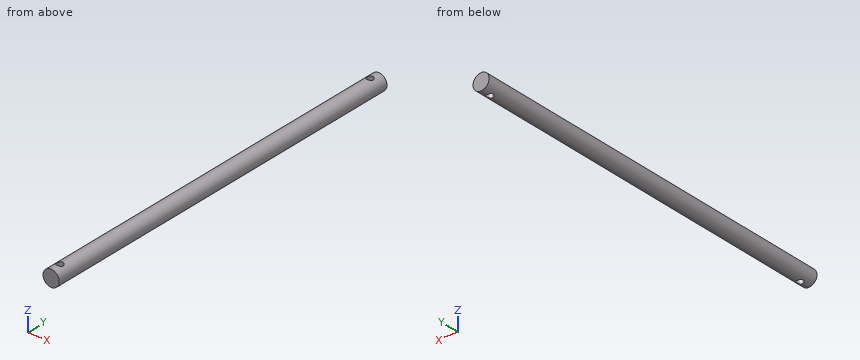
from build123d import *

# Parameters (mm, degrees)
CROQUIS1_R                 = 5
SALIENTE_EXTRUIR1_DEPTH    = 339
CROQUIS2_R                 = 6.894742802
CORTAR_EXTRUIR1_DEPTH      = 99.5
CORTAR_EXTRUIR2_DEPTH      = 10
CORTAR_EXTRUIR2_DEPTH_BACK = 10
CROQUIS3_R                 = 2
CORTAR_EXTRUIR3_DEPTH      = 10
CORTAR_EXTRUIR3_DEPTH_BACK = 10
CROQUIS4_R                 = 2


with BuildPart() as part:
    # Croquis1 → Saliente-Extruir1 (new body)
    with BuildSketch(Plane(origin=(0, 0, 0), x_dir=(1, 0, 0), z_dir=(0, 1, 0))):
        with Locations(Location((0, 0, 0), (0, 0, 270))):
            Circle(CROQUIS1_R)
    extrude(amount=SALIENTE_EXTRUIR1_DEPTH)

    # Croquis2 → Cortar-Extruir1 (cut)
    with BuildSketch(Plane(origin=(0, 339, 0), x_dir=(1, 0, 0), z_dir=(0, 1, 0))):
        Circle(CROQUIS2_R)
    extrude(amount=-CORTAR_EXTRUIR1_DEPTH, mode=Mode.SUBTRACT)

    # Croquis3 → Cortar-Extruir2 (cut, two sides: drawn at the far end of the back side and taken through both)
    with BuildSketch(Plane.XY.offset(-CORTAR_EXTRUIR2_DEPTH_BACK)):
        with Locations(Location((0, 6.5, 0), (0, 0, 90.000000001))):
            Circle(CROQUIS3_R)
    extrude(amount=CORTAR_EXTRUIR2_DEPTH + CORTAR_EXTRUIR2_DEPTH_BACK, mode=Mode.SUBTRACT)

    # Croquis4 → Cortar-Extruir3 (cut, two sides: drawn at the far end of the back side and taken through both)
    with BuildSketch(Plane.XY.offset(-CORTAR_EXTRUIR3_DEPTH_BACK)):
        with Locations(Location((0, 233, 0), (0, 0, 90.000000001))):
            Circle(CROQUIS4_R)
    extrude(amount=CORTAR_EXTRUIR3_DEPTH + CORTAR_EXTRUIR3_DEPTH_BACK, mode=Mode.SUBTRACT)


solid = part.part
Input: part model. Units: mm. Frame: model coordinates. Coordinates: 2 decimals unless noted, no trailing zeros. Write each loop counter-clockwise with the first axis right and the second up, starting at its lowest first coordinate (ties: lowest second). Pieces come first, ordered by that corner, then holes. Notation, with made-up numbers: M -3,-32.75 L 8,-32.75 A16 cw 8,-2.75 Z; hole C 44.5,-1.75 d4. An arc over 180 degrees is marked long. Answer as a JSON object with one key per item and string values. Group by question number.
(1) Section B-B on z = 2. Output: boundary loops of the cut face in (x, y), plus the area to 3 significant figures.
(2) Contact query for flat-ended pins moving along their axis: P1, Ø2, axis at x = 4, y = 76, coming from the +Z side; P2, Ø3.5, axis at x = 0, y = 233, coming from the -Z side; P3, Ø1, axis at x = 1.5, y = 197, coming from the +Z side. Output: stop coordinate, or through.
(3) Ray query, line 1 along Y through (x, z) = (0, 1.5); line 2 along Y through (x, z) = (0.5, -3); line 3 along Z through (x, y) = (0.5, 126). Return the intervals inside material, ascending. Write a range as [from, to].
(4) Section A-A on x = 0. Output: boundary loops of the cut face in (y, z), plus the area to 4 significant figures.
(5) Section C-C on y = 116. Output: boundary loops of the cut face in (x, z).
(6) Section D-D on y = 233. Output: boundary loops of the cut face in (x, z).
Result set:
{
 "1": {"outline": "M -4.58,0 L 4.58,0 L 4.58,239.5 L -4.58,239.5 Z; hole C 0,6.5 d4; hole C 0,233 d4", "area": "2,170 mm2"},
 "2": {"P1": "stops at z = 4", "P2": "passes through", "P3": "stops at z = 4.9"},
 "3": {"line 1": "y = [0, 4.5], [8.5, 231], [235, 239.5]", "line 2": "y = [0, 4.56], [8.44, 231.06], [234.94, 239.5]", "line 3": "z = [-4.97, 4.97]"},
 "4": {"outline": "M 0,-5 L 4.5,-5 L 4.5,5 L 0,5 Z; M 8.5,-5 L 231,-5 L 231,5 L 8.5,5 Z; M 235,-5 L 239.5,-5 L 239.5,5 L 235,5 Z", "area": "2,315 mm2"},
 "5": {"outline": "C 0,0 d10"},
 "6": {"outline": "M -2,-4.58 L -2,4.58 A5 ccw Z; M 2,-4.58 A5 ccw 2,4.58 Z"}
}
